```python
from build123d import *

# Parameters (mm, degrees)
SKETCH1_W            = 27.578431842
SKETCH1_H            = 27.578431842
SKETCH1_R            = 0.875
BOSS_EXTRUDE1_DEPTH  = 5
SKETCH2_W            = 5
SKETCH2_H            = 27.578431842
BOSS_EXTRUDE2_DEPTH  = 30
CUT_EXTRUDE2_DEPTH   = 10
SKETCH5_R            = 1.5
CUT_EXTRUDE3_DEPTH   = 24
FILLET1_R            = 8
FILLET2_R            = 8
SKETCH6_W            = 10
SKETCH6_H            = 10
CUT_EXTRUDE5_DEPTH   = 7
SKETCH7_R            = 3
CUT_EXTRUDE6_DEPTH   = 7
SKETCH8_W            = 3.789215921
SKETCH8_H            = 5
BOSS_EXTRUDE3_DEPTH  = 5
CUT_EXTRUDE7_DEPTH   = 25
SKETCH10_W           = 27.578431842
SKETCH10_H           = 5
BOSS_EXTRUDE4_DEPTH  = 11.61
BOSS_EXTRUDE5_DEPTH  = 5
BOSS_EXTRUDE9_DEPTH  = 5
SKETCH18_W           = 5
SKETCH18_H           = 7
BOSS_EXTRUDE10_DEPTH = 5
CUT_EXTRUDE9_DEPTH   = 59
SKETCH20_R           = 2
CUT_EXTRUDE10_DEPTH  = 10
BOSS_EXTRUDE11_DEPTH = 5


with BuildPart() as part:
    # Sketch1 → Boss-Extrude1 (new body)
    with BuildSketch(Plane(origin=(0, 0, 0), x_dir=(1, 0, 0), z_dir=(0, 1, 0))):
        with Locations((13.789215921, 13.789215921)):
            Rectangle(SKETCH1_W, SKETCH1_H)
        with Locations((2.032931996, 2.032931996)):
            Circle(SKETCH1_R, mode=Mode.SUBTRACT)
        with Locations((25.545499846, 25.545499846)):
            Circle(SKETCH1_R, mode=Mode.SUBTRACT)
        with Locations((2.032931996, 25.545499846)):
            Circle(SKETCH1_R, mode=Mode.SUBTRACT)
        with Locations((25.545513651, 2.032918191)):
            Circle(SKETCH1_R, mode=Mode.SUBTRACT)
    extrude(amount=BOSS_EXTRUDE1_DEPTH)

    # Sketch2 → Boss-Extrude2 (add)
    with BuildSketch(Plane(origin=(0, 5, 0), x_dir=(1, 0, 0), z_dir=(0, 1, 0))):
        with Locations((21.289215921, 13.789215921)):
            Rectangle(SKETCH2_W, SKETCH2_H)
        with Locations((6.289215921, 13.789215921)):
            Rectangle(SKETCH2_W, SKETCH2_H)
    extrude(amount=BOSS_EXTRUDE2_DEPTH)

    # Sketch4 → Cut-Extrude2 (cut)
    with BuildSketch(Plane.ZY.offset(-3.789215921)):
        with BuildLine():
            Line((-27.578431842, 11.509370995), (-27.578431842, 35))
            Line((-27.578431842, 35), (0, 35))
            Line((0, 35), (0, 11.509370995))
            ThreePointArc((0, 11.509370995), (-13.789215921, 15.656133254), (-27.578431842, 11.509370995))
        make_face()
    extrude(amount=-CUT_EXTRUDE2_DEPTH, mode=Mode.SUBTRACT)

    # Sketch5 → Cut-Extrude3 (cut)
    with BuildSketch(Plane(origin=(23.789215921, 0, 0), x_dir=(0, 0, -1), z_dir=(1, 0, 0))):
        with Locations((13.789215921, 29)):
            Circle(SKETCH5_R)
        with Locations((13.789215921, 11)):
            Circle(SKETCH5_R)
    extrude(amount=-CUT_EXTRUDE3_DEPTH, mode=Mode.SUBTRACT)

    # Fillet1
    fillet1_edges = [part.edges().sort_by_distance(p)[0] for p in [
        (21.289215921, 35, 0),
    ]]
    fillet(fillet1_edges, radius=FILLET1_R)

    # Fillet2
    fillet2_edges = [part.edges().sort_by_distance(p)[0] for p in [
        (21.289215921, 35, -27.578431842),
    ]]
    fillet(fillet2_edges, radius=FILLET2_R)

    # Sketch6 → Cut-Extrude5 (cut)
    with BuildSketch(Plane(origin=(0, 5, 0), x_dir=(1, 0, 0), z_dir=(0, 1, 0))):
        with Locations((13.789215921, 22.578431842)):
            Rectangle(SKETCH6_W, SKETCH6_H)
    extrude(amount=-CUT_EXTRUDE5_DEPTH, mode=Mode.SUBTRACT)

    # Sketch7 → Cut-Extrude6 (cut)
    with BuildSketch(Plane.XZ):
        with Locations((13.789215921, -13.789215921)):
            Circle(SKETCH7_R)
    extrude(amount=-CUT_EXTRUDE6_DEPTH, mode=Mode.SUBTRACT)

    # Sketch8 → Boss-Extrude3 (add)
    with BuildSketch(Plane(origin=(0, 5, 0), x_dir=(1, 0, 0), z_dir=(0, 1, 0))):
        with Locations((1.894607961, 19.170499846)):
            Rectangle(SKETCH8_W, SKETCH8_H)
        with Locations((25.683823882, 19.170499846)):
            Rectangle(SKETCH8_W, SKETCH8_H)
        with Locations((25.683823882, 8.407918191)):
            Rectangle(SKETCH8_W, SKETCH8_H)
        with Locations((1.894607961, 8.407918191)):
            Rectangle(SKETCH8_W, SKETCH8_H)
    extrude(amount=BOSS_EXTRUDE3_DEPTH)

    # Sketch9 → Cut-Extrude7 (cut)
    with BuildSketch(Plane.XY.offset(-5.907918191)):
        Polygon((0, 5), (3.789215921, 10), (0, 10), align=None)
        Polygon((23.789215921, 10), (27.578431842, 5), (27.578431842, 10), align=None)
    extrude(amount=-CUT_EXTRUDE7_DEPTH, mode=Mode.SUBTRACT)

    # Sketch10 → Boss-Extrude4 (add)
    with BuildSketch(Plane.ZY):
        with Locations((-13.789215921, 2.5)):
            Rectangle(SKETCH10_W, SKETCH10_H)
    extrude(amount=BOSS_EXTRUDE4_DEPTH)

    # Sketch11 → Boss-Extrude5 (add)
    with BuildSketch(Plane.ZY.offset(11.61)):
        Polygon((-32.758431842, 9.017116473), (-32.758431842, 0), (-27.578431842, 0), (0, 0), (25.24, 0), (25.24, 9.017116473), (25.24, 39), (16.24, 39), (16.24, 5), (0, 5), (-23.758431842, 5), (-23.758431842, 39), (-32.758431842, 39), align=None)
    extrude(amount=BOSS_EXTRUDE5_DEPTH)

    # Sketch17 → Boss-Extrude9 (add)
    with BuildSketch(Plane.ZY.offset(16.61)):
        Polygon((-23.758431842, 5), (-32.758431842, 5), (-32.758431842, 0), (25.24, 0), (25.24, 5), align=None)
    extrude(amount=BOSS_EXTRUDE9_DEPTH)

    # Sketch18 → Boss-Extrude10 (add)
    with BuildSketch(Plane(origin=(0, 5, 0), x_dir=(1, 0, 0), z_dir=(0, 1, 0))):
        with Locations((-19.11, 28.258431842)):
            Rectangle(SKETCH18_W, SKETCH18_H)
        with Locations((-19.11, -20.74)):
            Rectangle(SKETCH18_W, SKETCH18_H)
    extrude(amount=BOSS_EXTRUDE10_DEPTH)

    # Sketch19 → Cut-Extrude9 (cut)
    with BuildSketch(Plane.XY.offset(24.24)):
        Polygon((-21.61, 5), (-21.61, 10), (-16.61, 10), align=None)
    extrude(amount=-CUT_EXTRUDE9_DEPTH, mode=Mode.SUBTRACT)

    # Sketch20 → Cut-Extrude10 (cut)
    with BuildSketch(Plane(origin=(-11.61, 0, 0), x_dir=(0, 0, -1), z_dir=(1, 0, 0))):
        with Locations((-21.738681897, 34.501289775)):
            Circle(SKETCH20_R)
        with Locations((-21.785282729, 23.501291949)):
            Circle(SKETCH20_R)
        with Locations((29.260801868, 23.498896595)):
            Circle(SKETCH20_R)
        with Locations((29.261318047, 34.498896583)):
            Circle(SKETCH20_R)
    extrude(amount=-CUT_EXTRUDE10_DEPTH, mode=Mode.SUBTRACT)

    # Sketch21 → Boss-Extrude11 (add)
    with BuildSketch(Plane(origin=(0, 5, 0), x_dir=(1, 0, 0), z_dir=(0, 1, 0))):
        Polygon((-11.61, -25.24), (27.578431842, 0), (-11.61, 0), align=None)
        Polygon((-11.61, 32.758431842), (8.789215921, 27.578431842), (-11.61, 27.578431842), align=None)
    extrude(amount=-BOSS_EXTRUDE11_DEPTH)


solid = part.part
```
Model file for the job. Use its own axes, mm. A direction names the side the tool comes from. Round coordinates to 2 decimals unless told otherwise and drop trailing zeros. Write each loop counter-clockwise with the first axis right and the second up, starting at its lowest first coordinate (ties: lowest second). Pieces come first, ordered by that corner, then holes. Notation, with made-up numbers: M 16,82 L 32,82 A35 cw 32,114 Z; hole C 26.5,-33 d7. An arc over 180 degrees is marked long. Put each result on its own line as item: value.
Item 1: Cut at A-A (y = 17). List the corners of the cut face in (x, z), and give its area (3 significant figures).
Responses:
outline: M -16.61,-32.76 L -11.61,-32.76 L -11.61,-23.76 L -16.61,-23.76 Z; M -16.61,16.24 L -11.61,16.24 L -11.61,25.24 L -16.61,25.24 Z; M 18.79,-27.58 L 23.79,-27.58 L 23.79,0 L 18.79,0 Z
area: 228 mm²
Item 2: Mould opens along Y. For faces 5 (the flat face through (-18, 6, 17.24)), 6 (the flat face through (26, 5, -14)), 7 (the cylindrical face through (-14.08, 33.74, 19.89)) say: +Y half, -Y half, draft (parallel to the pull), parting line (faces both ways), or undercut.
Responses:
face 5: draft
face 6: +Y half
face 7: undercut
Item 3: Flat gauge pins, fed straight in: P1, Ø5, axis at y = 17, z = -16.5, coming from the +X side; P2, Ø4, axis at x = 21.5, z = -20.5, coming from the +Y side; P3, Ø4, axis at x = 20.5, y = 21, coming from the +Z side; P4, Ø3, axis at y = 34, z = 0.5, coming from the +X side. Where does each tip first touch, or does it go through?
Responses:
P1: x = 23.79
P2: y = 35
P3: z = 0
P4: through
Item 4: Cut at D-D (x = 15). List the corners of the cut face in (y, z).
Responses:
outline: M 0,-17.58 L 5,-17.58 L 5,-16.53 L 0,-16.53 Z; M 0,-11.04 L 5,-11.04 L 5,8.1 L 0,8.1 Z
Item 5: Probe L1, parallel to Y at x = -14.5, z = 22; L2, parallel to Z at x = 20, y = 18.5; L3, parallel to Y at x = -0.5, z = -2. List the from-to ranges inside material, lowest first. Write a range as from..to.
Responses:
L1: 0..21.51, 25.49..32.52, 36.48..39
L2: -27.58..0
L3: 0..5
Item 6: Cut at B-B (z = 21.5). List the corners of the cut face in (x, y), and give its area (3 significant figures).
Responses:
outline: M -21.61,0 L -5.8,0 L -5.8,5 L -11.61,5 L -11.61,21.52 L -16.61,21.52 L -16.61,10 L -21.61,5 Z; M -16.61,25.48 L -11.61,25.48 L -11.61,32.52 L -16.61,32.52 Z; M -16.61,36.49 L -11.61,36.49 L -11.61,39 L -16.61,39 Z
area: 222 mm²
Item 7: Cut at C-C (y = 29). List the corners of the cut face in (x, z).
Responses:
outline: M -16.61,-32.76 L -11.61,-32.76 L -11.61,-23.76 L -16.61,-23.76 Z; M -16.61,16.24 L -11.61,16.24 L -11.61,25.24 L -16.61,25.24 Z; M 18.79,-27.32 L 23.79,-27.32 L 23.79,-15.29 L 18.79,-15.29 Z; M 18.79,-12.29 L 23.79,-12.29 L 23.79,-0.25 L 18.79,-0.25 Z
Item 8: Tool access for faces 1 (the flat face through (-11.61, 22, 20)), 2 (the flat face through (25, 7, -5.908)), 3 (the flat face through (-18, 6, -31.758)), 4 (the flat face through (3, 6, -16.67)): list every direction of +Z, -Z, +X, -X, +Y, -Y with a clear straight run to the whole face (end or side of a thin tool).
Responses:
face 1: +Z, -Z, +X, +Y
face 2: +Z, +X, +Y
face 3: -Z, -X, +Y
face 4: -X, +Y
